from build123d import *

# Parameters (mm, degrees)
F1_DEPTH     = 2
F2_W         = 5.5
F2_H         = 2.5
F3_DEPTH     = 18
F6_DEPTH     = 1.34
F7_D         = 4
F7_DEPTH     = 4
F7_START     = 3.5
F7_TIP       = 1.2017212381
F8_DEPTH     = 3.5
F9_T4_DEPTH  = 11.4580124596
F9_S5_R      = 7.5
F9_T6_DEPTH  = 7
F9_T12_DEPTH = 11.4580124596
F9_S13_R     = 7.5
F9_T14_DEPTH = 7
F9_T20_DEPTH = 11.4580124596
F9_S21_R     = 7.5
F9_T22_DEPTH = 7
F10_SIZE     = 0.4


# Not quite as in the source:
# - a fillet or chamfer that OpenCascade refuses, or shapes differently, is made with other operations: its cross-section is extruded or revolved along the edge and cut away or added


with BuildPart() as f1:
    # F0 (on Top) → F1 (new body)
    with BuildSketch(Plane.XY):
        with BuildLine():
            ThreePointArc((-3.5, 6.6332495807), (-3.8729833462, -6.4226162893), (7.5, 0))
            ThreePointArc((7.5, 0), (6.4226162893, 3.8729833462), (3.5, 6.6332495807))
            Line((3.5, 6.6332495807), (-3.5, 6.6332495807))
        make_face()
        with BuildLine():
            ThreePointArc((1.1874342087, 2.2), (2.146926352, 1.2809009482), (2.5, 0))
            ThreePointArc((2.5, 0), (-1.2809009482, -2.146926352), (-1.1874342087, 2.2))
            ThreePointArc((-1.1874342087, 2.2), (0, 2.5), (1.1874342087, 2.2))
        make_face(mode=Mode.SUBTRACT)
        with BuildLine():
            Line((-3.5, 6.6332495807), (3.5, 6.6332495807))
            ThreePointArc((3.5, 6.6332495807), (0, 7.5), (-3.5, 6.6332495807))
        make_face()
    extrude(amount=F1_DEPTH)

    # F2 (on face) → F3 (join)
    with BuildSketch(Plane.XY.offset(2)):
        with BuildLine():
            ThreePointArc((-3.5, 6.6332495807), (-3.8729833462, -6.4226162893), (7.5, 0))
            ThreePointArc((7.5, 0), (6.4226162893, 3.8729833462), (3.5, 6.6332495807))
            Line((3.5, 6.6332495807), (-3.5, 6.6332495807))
        make_face()
        with BuildLine():
            ThreePointArc((1.1874342087, 2.2), (2.146926352, 1.2809009482), (2.5, 0))
            ThreePointArc((2.5, 0), (-1.2809009482, -2.146926352), (-1.1874342087, 2.2))
            ThreePointArc((-1.1874342087, 2.2), (0, 2.5), (1.1874342087, 2.2))
        make_face(mode=Mode.SUBTRACT)
        with Locations((0, 4.3832495807)):
            Rectangle(F2_W, F2_H, mode=Mode.SUBTRACT)
        with BuildLine():
            Line((-1.1874342087, 2.2), (1.1874342087, 2.2))
            ThreePointArc((1.1874342087, 2.2), (0, 2.5), (-1.1874342087, 2.2))
        make_face()
    extrude(amount=F3_DEPTH)

    # F5 (on face) → F6 (cut)
    with BuildSketch(Plane(origin=(0, 6.6332495807, 0), x_dir=(-1, 0, 0), z_dir=(0, 1, 0))):
        with BuildLine():
            Line((1.7, 20), (-1.7, 20))
            Line((-1.7, 20), (-1.7, 16.0535653753))
            ThreePointArc((-1.7, 16.0535653753), (0, 17), (1.7, 16.0535653753))
            Line((1.7, 16.0535653753), (1.7, 20))
        make_face()
        Polygon((-1.7, 3.8314954576), (-1.7, 2), (1.7, 2), (1.7, 3.8314954576), (0, 2.85), align=None)
        with BuildLine():
            Line((1.7, 15), (-1.7, 15))
            Line((-1.7, 15), (-1.7, 13.9464346247))
            ThreePointArc((-1.7, 13.9464346247), (0, 13), (1.7, 13.9464346247))
            Line((1.7, 13.9464346247), (1.7, 15))
        make_face()
        with BuildLine():
            Line((-1.7, 15), (-2, 15))
            ThreePointArc((-2, 15), (-1.9235384062, 14.4522774425), (-1.7, 13.9464346247))
            Line((-1.7, 13.9464346247), (-1.7, 15))
        make_face()
        with BuildLine():
            ThreePointArc((-1.7, 16.0535653753), (-1.9235384062, 15.5477225575), (-2, 15))
            Line((-2, 15), (-1.7, 15))
            Line((-1.7, 15), (-1.7, 16.0535653753))
        make_face()
        with BuildLine():
            Line((1.7, 16.0535653753), (1.7, 15))
            Line((1.7, 15), (2, 15))
            ThreePointArc((2, 15), (1.9235384062, 15.5477225575), (1.7, 16.0535653753))
        make_face()
        with BuildLine():
            Line((2, 15), (1.7, 15))
            Line((1.7, 15), (1.7, 13.9464346247))
            ThreePointArc((1.7, 13.9464346247), (1.9235384062, 14.4522774425), (2, 15))
        make_face()
        with BuildLine():
            Line((-1.7, 16.0535653753), (-1.7, 15))
            Line((-1.7, 15), (1.7, 15))
            Line((1.7, 15), (1.7, 16.0535653753))
            ThreePointArc((1.7, 16.0535653753), (0, 17), (-1.7, 16.0535653753))
        make_face()
        with BuildLine():
            Line((-1.7, 6), (-1.7, 4.9464346247))
            ThreePointArc((-1.7, 4.9464346247), (0, 4), (1.7, 4.9464346247))
            Line((1.7, 4.9464346247), (1.7, 6))
            Line((1.7, 6), (-1.7, 6))
        make_face()
        with BuildLine():
            ThreePointArc((-2, 6), (-1.9235384062, 5.4522774425), (-1.7, 4.9464346247))
            Line((-1.7, 4.9464346247), (-1.7, 6))
            Line((-1.7, 6), (-2, 6))
        make_face()
        with BuildLine():
            Line((-1.7, 7.0535653753), (-1.7, 6))
            Line((-1.7, 6), (1.7, 6))
            Line((1.7, 6), (1.7, 7.0535653753))
            ThreePointArc((1.7, 7.0535653753), (0, 8), (-1.7, 7.0535653753))
        make_face()
        with BuildLine():
            Line((1.7, 7.0535653753), (1.7, 6))
            Line((1.7, 6), (2, 6))
            ThreePointArc((2, 6), (1.9235384062, 6.5477225575), (1.7, 7.0535653753))
        make_face()
        with BuildLine():
            Line((1.7, 6), (1.7, 4.9464346247))
            ThreePointArc((1.7, 4.9464346247), (1.9235384062, 5.4522774425), (2, 6))
            Line((2, 6), (1.7, 6))
        make_face()
        with BuildLine():
            ThreePointArc((-1.7, 7.0535653753), (-1.9235384062, 6.5477225575), (-2, 6))
            Line((-2, 6), (-1.7, 6))
            Line((-1.7, 6), (-1.7, 7.0535653753))
        make_face()
        with BuildLine():
            Line((-1.7, 4.9464346247), (-1.7, 3.8314954576))
            Line((-1.7, 3.8314954576), (0, 2.85))
            Line((0, 2.85), (1.7, 3.8314954576))
            Line((1.7, 3.8314954576), (1.7, 4.9464346247))
            ThreePointArc((1.7, 4.9464346247), (0, 4), (-1.7, 4.9464346247))
        make_face()
        with BuildLine():
            ThreePointArc((1.7, 13.9464346247), (0, 13), (-1.7, 13.9464346247))
            Line((-1.7, 13.9464346247), (-1.7, 8.1685045424))
            Line((-1.7, 8.1685045424), (0, 9.15))
            Line((0, 9.15), (1.7, 8.1685045424))
            Line((1.7, 8.1685045424), (1.7, 13.9464346247))
        make_face()
        with BuildLine():
            Line((-1.7, 8.1685045424), (-1.7, 7.0535653753))
            ThreePointArc((-1.7, 7.0535653753), (0, 8), (1.7, 7.0535653753))
            Line((1.7, 7.0535653753), (1.7, 8.1685045424))
            Line((1.7, 8.1685045424), (0, 9.15))
            Line((0, 9.15), (-1.7, 8.1685045424))
        make_face()
    extrude(amount=-F6_DEPTH, mode=Mode.SUBTRACT)

    # F7
    # its depths count from where the whole tool has entered the part; down to there all is cleared
    with Locations(Plane(origin=(0, 6.6332495807, 0), x_dir=(-1, 0, 0), z_dir=(0, 1, 0)).offset(-F7_START)):
        with Locations((0, 6), (0, 15)):
            Hole(F7_D / 2, depth=F7_DEPTH)
            with Locations((0, 0, -(F7_DEPTH + F7_TIP / 2))):  # 118° drill point
                Cone(0, F7_D / 2, F7_TIP, mode=Mode.SUBTRACT)

    # F5 (on face) → F8 (join)
    with BuildSketch(Plane(origin=(0, 6.6332495807, 0), x_dir=(-1, 0, 0), z_dir=(0, 1, 0))):
        Polygon((-3.5, 6), (-3.5, 2), (-1.7, 2), (-1.7, 3.8314954576), (-2.7279800219, 4.425), (-2.7279800219, 6), align=None)
        Polygon((-1.7, 3.8314954576), (-1.7, 2), (1.7, 2), (1.7, 3.8314954576), (0, 2.85), align=None)
        Polygon((1.7, 3.8314954576), (1.7, 2), (3.5, 2), (3.5, 6), (2.7279800219, 6), (2.7279800219, 4.425), align=None)
    extrude(amount=-F8_DEPTH)

    # F9: chamfer of 0.86675 on 1 edges, made by hand


with BuildPart() as f9_tool2:
    # F9_s3 → F9_t4 (new body)
    with BuildSketch(Plane.YZ.offset(5.7290062298)):
        Polygon((6.6332495807, 2.86675), (7.4999995807, 2), (6.6332495807, 2), align=None)
    extrude(amount=-F9_T4_DEPTH)

    # F9_s5 → F9_t6 (intersect, symmetric)
    with BuildSketch(Plane.XY.offset(2.4)):
        Circle(F9_S5_R)
    extrude(amount=F9_T6_DEPTH, both=True, mode=Mode.INTERSECT)

    split(bisect_by=Plane(origin=(-1.2340862004, 0, 2.1375), x_dir=(0, 1, 0), z_dir=(0.5, 0, -0.8660254038)), keep=Keep.TOP)

    split(bisect_by=Plane(origin=(1.2340862004, 0, 2.1375), x_dir=(0, 1, 0), z_dir=(0.5, 0, 0.8660254038)), keep=Keep.TOP)


with BuildPart() as f1_1:
    add(f1.part)

    # F9_t1: union F9_tool2
    add(f9_tool2.part)


with BuildPart() as f9_tool10:
    # F9_s11 → F9_t12 (new body)
    with BuildSketch(Plane.YZ.offset(5.7290062298)):
        Polygon((6.6332495807, 2.86675), (7.4999995807, 2), (6.6332495807, 2), align=None)
    extrude(amount=-F9_T12_DEPTH)

    # F9_s13 → F9_t14 (intersect, symmetric)
    with BuildSketch(Plane.XY.offset(2.4)):
        Circle(F9_S13_R)
    extrude(amount=F9_T14_DEPTH, both=True, mode=Mode.INTERSECT)

    split(bisect_by=Plane(origin=(-1.2340862004, 0, 2.1375), x_dir=(0, 1, 0), z_dir=(0.5, 0, -0.8660254038)), keep=Keep.TOP)

    split(bisect_by=Plane(origin=(1.2340862004, 0, 2.1375), x_dir=(0, 1, 0), z_dir=(-0.5, 0, -0.8660254038)), keep=Keep.TOP)


with BuildPart() as f1_2:
    add(f1_1.part)

    # F9_t9: union F9_tool10
    add(f9_tool10.part)


with BuildPart() as f9_tool18:
    # F9_s19 → F9_t20 (new body)
    with BuildSketch(Plane.YZ.offset(5.7290062298)):
        Polygon((6.6332495807, 2.86675), (7.4999995807, 2), (6.6332495807, 2), align=None)
    extrude(amount=-F9_T20_DEPTH)

    # F9_s21 → F9_t22 (intersect, symmetric)
    with BuildSketch(Plane.XY.offset(2.4)):
        Circle(F9_S21_R)
    extrude(amount=F9_T22_DEPTH, both=True, mode=Mode.INTERSECT)

    split(bisect_by=Plane(origin=(-1.2340862004, 0, 2.1375), x_dir=(0, 1, 0), z_dir=(-0.5, 0, 0.8660254038)), keep=Keep.TOP)

    split(bisect_by=Plane(origin=(1.2340862004, 0, 2.1375), x_dir=(0, 1, 0), z_dir=(-0.5, 0, -0.8660254038)), keep=Keep.TOP)


with BuildPart() as f1_3:
    add(f1_2.part)

    # F9_t17: union F9_tool18
    add(f9_tool18.part)

    # F10
    f10_edges = [f1_3.edges().sort_by_distance(p)[0] for p in [
        (-7.5, 0, 0),
        (-1.187434, -2.2, 0),
        (0, -2.5, 20),
        (0, -7.5, 20),
        (0, 3.13325, 20),
        (2.75, 4.38325, 20),
        (2.225, 5.63325, 20),
        (-2.225, 5.63325, 20),
        (-2.75, 4.38325, 20),
    ]]
    chamfer(f10_edges, length=F10_SIZE)


solid = f1_3.part
CAD build for the part. Positions are in the model's coordinates, mm. A direction names the side the tool comes from. Round coordinates to 2 decimals unless told otherwise and drop trailing zeros. Loops run counter-clockwise (first coordinate to the right, second up) from the corner with the lowest first, then second, coordinate; pieces in that order, holes last.
(1) Cut at C-C (z = 15.5). Give the cut face in (x, y), plus the area to 3 significant figures.
(2) Cut at B-B (x = 0.5). State how many separate pieces and enclosed holes the cut face has, plus the area to 3 significant figures.
(3) Drop flat-ended pins along their axis: pin 1 (2 mm diameter, centred on x = 2, z = 16, fed in from +Y); pin 2 (3.5 mm diameter, centred on x = 0, z = 6, fed in from +Y); pin 3 (4 mm diameter, centred on x = 4.5, z = 2.5, fed in from -Y). Give the stop position or say it passes through.
(4) Which spindle directions (+Z, -Z, +X, -X, +Y, -Y) get a long thin tool onto all of the face, cutting with end or side? Do faces 1 (the flat face through (-3, 6.633, 11)), 2 (the flat face through (-2.728, 4, 5)), 3 (the flat face through (-1.7, 6, 4)), 4 (the cylindrical face through (-1.6, 2.5, 13.8)), 5 (the flat face through (0, 2.2, 3)). Say none if no direction does.
(5) Wall check: line 1 along Z through (x, y) = (0, 2.3); line 2 along Z through (x, y) = (-1.5, 2.25); line 3 along Y through (x, z) = (-2, 15.75). Give the ranges that are in metal, low to high.
(6) Cut at A-A (z = 18.75). Give the cut face in (x, y).
(7) Two-plate mould, pull along Y, no slides. Class faces 6 (the flat face through (1.7, 6, 11)), 7 (the flat face through (2, 5.633, 12)), 8 (the flat face through (0, 7, 2.5)): +Y half, -Y half, draft (parallel to the pull), parting line (faces both ways), or undercut.
Findings below:
1. outline: (-3.5, 6.63) arc R7.5 ccw (long way) to (3.5, 6.63) - (1.94, 6.63) - (1.94, 5.63) - (2.75, 5.63) - (2.75, 3.13) - (1.94, 3.13) - (1.94, 1.58) arc R2.5 cw (long way) to (-1.94, 1.58) - (-1.94, 3.13) - (-2.75, 3.13) - (-2.75, 5.63) - (-1.94, 5.63) - (-1.94, 6.63) - close
1. area: 132 mm2
2. separate pieces: 4
2. enclosed holes: 0
2. area: 124 mm2
3. pin 1: stops at y = 6.63
3. pin 2: stops at y = -1.79
3. pin 3: stops at y = -7.07
4. face 1: +Z, +X, -X, +Y
4. face 2: +Z
4. face 3: +Z, +Y
4. face 4: +Y
4. face 5: +Z, -Z
5. line 1: z = 2 to 4, 8 to 13, 17 to 20
5. line 2: z = 0.2 to 4.68, 7.32 to 13.68, 16.32 to 20
5. line 3: y = -7.23 to -1.5, 1.5 to 3.13, 5.63 to 6.63
6. outline: (-3.5, 6.63) arc R7.5 ccw (long way) to (3.5, 6.63) - (1.7, 6.63) - (1.7, 5.63) - (2.75, 5.63) - (2.75, 3.13) - (-2.75, 3.13) - (-2.75, 5.63) - (-1.7, 5.63) - (-1.7, 6.63) - close; hole (-1.19, 2.2) arc R2.5 ccw (long way) to (1.19, 2.2) - close
7. face 6: draft
7. face 7: undercut
7. face 8: +Y half
